Geometry: final body of the model. Coordinates: model frame, mm. A direction names the side the tool comes from. Give positions to 0.01 mm unless a question says otherwise; leave off trailing zeros. Order: outer loops, then holes, each group sorted by start corner. A loop starts at its lowest first (then second) coordinate and runs counter-clockwise, first axis right, second up. Notation, with made-up numbers: (-6.75, -32) -> (17.25, -32) arc R27 ccw to (17.25, -3) -> close; hole circle Ø3 at (9, -21). An arc over 180 degrees is marked (long way). One line per item, written item: value. Start each with the question number.
```python
from build123d import *

# Parameters (mm, degrees)
F0_R     = 9
F1_DEPTH = 1.5
F2_R     = 11
F2_R_2   = 9
F3_DEPTH = 23
F6_R     = 1


with BuildPart() as f1:
    # F0 (on Top) → F1 (new body)
    with BuildSketch(Plane.XY):
        Circle(F0_R)
    extrude(amount=F1_DEPTH)

    # F2 (on Top) → F3 (join)
    with BuildSketch(Plane.XY):
        Circle(F2_R)
        Circle(F2_R_2, mode=Mode.SUBTRACT)
    extrude(amount=F3_DEPTH)

    # F4 (on Front) → F5 (revolve, cut)
    with BuildSketch(Plane.XZ):
        with BuildLine():
            ThreePointArc((8.997346, 20.502327), (8.82057, 20.07555), (9.247346, 20.252327))
            ThreePointArc((9.247346, 20.252327), (9.174123, 20.429104), (8.997346, 20.502327))
        make_face()
    revolve(axis=Axis((0, 0, 0), (0, 0, -1)), mode=Mode.SUBTRACT)

    # F6
    f6_edges = [f1.edges().sort_by_distance(p)[0] for p in [
        (-9, 0, 1.5),
        (-11, 0, 0),
    ]]
    fillet(f6_edges, radius=F6_R)


solid = f1.part
```
1. Pin query (flat end, axial travel): P1, Ø10, axis at x = -4.5, z = 9.5, coming from the -Y side; P2, Ø2, axis at x = -4, y = -5, coming from the +Z side; P3, Ø2, axis at x = -3.5, z = 2.5, coming from the -Y side; P4, Ø1, axis at x = 1, z = 4, coming from the +Y side. Return the tip coordinate at first contact, or that it passes through.
2. Access query for faces 4 (the flat face through (0, 0, 0)), 5 (the cylindrical face through (-1.172, 8.923, 21.734)). Directions: +Z, -Z, +X, -X, +Y, -Y. A direction counts if a zero-diameter tool reaches every point of the face in a straight line with its end or side. Return the directions, or none.
3. Material intervals for L1, parallel to Y at x = 0, z = 22.25; L2, parallel to Z at x = -7.5, y = 3; L3, parallel to Y at x = -7.75, z = 11.5, sorted ascending. Write a range as [from, to].
4. Cut plane A-A, the plane z = 6. Return loops of the section in (x, y), then the cut area to 3 significant figures.
5. Draft query along X for faces 1 (the flat face through (2, -9, 23)), 2 (the flat face through (0, 0, 1.5)), 3 (the cylindrical face through (-2.38, -10.74, 11.85)). Return one class per face: pulls with the +X half, pulls with the -X half, needs draft (parallel to the pull), parting line crosses it, or undercut.
Answers follow:
1. P1: stops at y = -11
1. P2: stops at z = 1.5
1. P3: stops at y = -10.71
1. P4: stops at y = 10.99
2. face 4: -Z, +X, -X, +Y, -Y
2. face 5: +Z
3. L1: y = [-11, -9], [9, 11]
3. L2: z = [0, 1.5]
3. L3: y = [-7.81, -4.58], [4.58, 7.81]
4. outline: circle Ø22 at (0, 0); hole circle Ø18 at (0, 0)
4. area: 126 mm²
5. face 1: needs draft
5. face 2: undercut
5. face 3: parting line crosses it
